```python
from build123d import *

# Parameters (mm, degrees)
SKETCH1_R           = 11.049
BOSS_EXTRUDE1_DEPTH = 19.05
SKETCH2_R           = 12.7
BOSS_EXTRUDE2_DEPTH = 6.35
SKETCH3_R           = 5.5
CUT_EXTRUDE1_DEPTH  = 32.108519733
SKETCH4_R           = 11.1125
CUT_EXTRUDE2_DEPTH  = 5.5372
CHAMFER1_SIZE       = 0.299999908


with BuildPart() as part:
    # Sketch1 → Boss-Extrude1 (new body)
    with BuildSketch(Plane(origin=(0, 0, 0), x_dir=(1, 0, 0), z_dir=(0, 1, 0))):
        with Locations(Location((0, 0, 0), (0, 0, 90))):
            Circle(SKETCH1_R)
    extrude(amount=BOSS_EXTRUDE1_DEPTH)

    # Sketch2 → Boss-Extrude2 (add)
    with BuildSketch(Plane.XZ):
        with Locations(Location((0, 0, 0), (0, 0, 270))):
            Circle(SKETCH2_R)
    extrude(amount=BOSS_EXTRUDE2_DEPTH)

    # Sketch3 → Cut-Extrude1 (cut, through all)
    with BuildSketch(Plane.XZ.offset(6.35)):
        with Locations(Location((0, 0, 0), (0, 0, 270))):
            Circle(SKETCH3_R)
    extrude(amount=-CUT_EXTRUDE1_DEPTH, mode=Mode.SUBTRACT)

    # Sketch4 → Cut-Extrude2 (cut)
    with BuildSketch(Plane.XZ.offset(6.35)):
        with Locations(Location((0, 0, 0), (0, 0, 270))):
            Circle(SKETCH4_R)
    extrude(amount=-CUT_EXTRUDE2_DEPTH, mode=Mode.SUBTRACT)

    # Chamfer1
    chamfer1_edges = [part.edges().sort_by_distance(p)[0] for p in [
        (0, 19.05, 5.5),
        (0, -6.35, 11.1125),
        (0, -0.8128, 5.5),
        (0, 19.05, 11.049),
        (0, 0, 12.7),
        (0, -6.35, 12.7),
    ]]
    chamfer(chamfer1_edges, length=CHAMFER1_SIZE)


solid = part.part
```
Part model, mm, in its own coordinate system. A direction names the side the tool comes from. Round coordinates to 2 decimals unless told otherwise and drop trailing zeros. Loops run counter-clockwise (first coordinate to the right, second up) from the corner with the lowest first, then second, coordinate; pieces in that order, holes last.
Item 1: Cut at D-D, the plane y = -2.25. Give the cut face in (x, z) (1 decimal), then the cut area to 3 significant figures.
Item 2: Mould opens along Z. For faces 4 (the face through (-7.47, 9.24, 8.14)), 5 (the face through (-5, -0.813, -5)), 6 (the face through (5, 19.05, -5)) say: +Z half, -Z half, draft (parallel to the pull), parting line (faces both ways), or undercut.
Item 3: Drill centre lines: line 1 (X direction, y = -2, z = 0); line 2 (X direction, y = 8.25, z = 0); line 3 (Y direction, x = 4.25, z = 9.5). Where is each one in solid material? Low to high.
Item 4: Cut at A-A, the plane x = 0. Give the cut face in (y, z), then the cut area to 3 significant figures.
Item 5: Drop flat-ended pins along their axis: P1, Ø12, axis at x = -6.5, y = 10, coming from the -Z side; P2, Ø5, axis at y = 9.5, z = -5, coming from the -X side; P3, Ø1.5, axis at y = -2.5, z = 1.5, coming from the +X side; P4, Ø6.5, axis at x = 0, z = 0, coming from the -Y side. Give the stop position or say it passes through.
Item 6: Cut at B-B, the plane z = 0. Give the cut face in (x, y).
Item 7: Cut at C-C, the plane y = 1.5. Give the cut face in (x, z).
Item 8: 3-axis set-ups, long thin cutter, end or side, ignore diameter. For faces 1 (the face through (-4, -6.35, -11)), 2 (the face through (9.37, -3.468, -5.974)), 3 (the face through (-1.8, 0, 11.1)): which of +Z, -Z, +X, -X, +Y, -Y reach the whole face in a straight line?
A:
1. outline: circle Ø25.4 at (0, 0); hole circle Ø22.2 at (0, 0)
1. area: 119 mm2
2. face 4: parting line
2. face 5: undercut
2. face 6: draft
3. line 1: x = -12.7 to -11.11, 11.11 to 12.7
3. line 2: x = -11.05 to -5.5, 5.5 to 11.05
3. line 3: y = -0.81 to 19.05
4. outline: (-6.35, -12.4) - (-6.05, -12.7) - (-0.3, -12.7) - (0, -12.4) - (0, -11.05) - (18.75, -11.05) - (19.05, -10.75) - (19.05, -5.8) - (18.75, -5.5) - (-0.51, -5.5) - (-0.81, -5.8) - (-0.81, -11.11) - (-6.05, -11.11) - (-6.35, -11.41) - close; (-6.35, 11.41) - (-6.05, 11.11) - (-0.81, 11.11) - (-0.81, 5.8) - (-0.51, 5.5) - (18.75, 5.5) - (19.05, 5.8) - (19.05, 10.75) - (18.75, 11.05) - (0, 11.05) - (0, 12.4) - (-0.3, 12.7) - (-6.05, 12.7) - (-6.35, 12.4) - close
4. area: 240 mm2
5. P1: stops at z = -11.04
5. P2: stops at x = -10.76
5. P3: stops at x = 12.68
5. P4: passes through
6. outline: (-12.7, -6.05) - (-12.4, -6.35) - (-11.41, -6.35) - (-11.11, -6.05) - (-11.11, -0.81) - (-5.8, -0.81) - (-5.5, -0.51) - (-5.5, 18.75) - (-5.8, 19.05) - (-10.75, 19.05) - (-11.05, 18.75) - (-11.05, 0) - (-12.4, 0) - (-12.7, -0.3) - close; (5.5, -0.51) - (5.8, -0.81) - (11.11, -0.81) - (11.11, -6.05) - (11.41, -6.35) - (12.4, -6.35) - (12.7, -6.05) - (12.7, -0.3) - (12.4, 0) - (11.05, 0) - (11.05, 18.75) - (10.75, 19.05) - (5.8, 19.05) - (5.5, 18.75) - close
7. outline: circle Ø22.1 at (0, 0); hole circle Ø11 at (0, 0)
8. face 1: +Z, -Z, +X, -X, -Y
8. face 2: -Y
8. face 3: +Y
